The listing builds one solid part. Answer for the finished solid, in the listing's coordinates (mm). A direction names the side the tool comes from. Round coordinates to 2 decimals unless told otherwise and drop trailing zeros. Write each loop counter-clockwise with the first axis right and the second up, starting at its lowest first coordinate (ties: lowest second). Pieces come first, ordered by that corner, then holes.
Item 1: Find section D-D on x = 98. Give the vertices of the cut face in (y, z), then the cut area to 3 significant figures.
Item 2: Find section B-B on z = 34. Give the vertices of the cut face in (x, y).
Item 3: Find section A-A on y = 181.5. Give the vertices of the cut face in (x, z).
Item 4: Each of these flat-tipped pins is pushed along its axis until it touches: pin 1 (13.5 mm diameter, centred on y = 1118.5, z = 44.5, fed in from -X); pin 2 (2 mm diameter, centred on x = 269.5, y = 349.5, fed in from +Z); pin 3 (8.5 mm diameter, centred on x = 2.5, y = 389, fed in from -Z). Where does it stop, or does it pass through?
Item 5: For a pull along X with two mould halves and no side action, classify faces 4 (the face through (419.562, 740, 41)), 5 (the face through (204.3, 1500, 17.7)), 6 (the face through (217, 740, 18.133)) as +X half, -X half, draft (parallel to the pull), parting line (faces both ways), or undercut.
Item 6: Find section C-C on y = 993. Give the vertices of the cut face in (x, z), then the cut area to 4 significant figures.
Item 7: A tool of negligible diameter and unlimited length cuts with its end or side. For faces 1 (the face through (418.062, 740, 41)), 2 (the face through (9.562, 740, 41)), 3 (the face through (11.062, 740, 42)), from which of +Z, -Z, +X, -X, +Y, -Y can it reach the whole face along a straight path? Write none if from no direction.
Item 8: Find the intervals of material crossed by probe 1 along X at (y, z) = (796.5, 39); probe 2 along X at (y, z) = (339, 56); probe 3 along Z at (x, y) = (278.5, 337), in increasing order.
```python
from build123d import *

# Parameters (mm, degrees)
F1_DEPTH = 1500
F2_W     = 20
F2_H     = 100
F3_DEPTH = 1.5


with BuildPart() as f1:
    # F0 (on Front) → F1 (new body)
    with BuildSketch(Plane.XZ):
        Polygon((9.56153, 65.133369), (9.56153, 16.633369), (419.56153, 16.633369), (419.56153, 65.133369), (402.56153, 65.133369), (402.56153, 63.633369), (418.06153, 63.633369), (418.06153, 18.133369), (11.06153, 18.133369), (11.06153, 66.633369), (-8.93847, 66.633369), (-8.93847, 51.633369), (-7.43847, 51.633369), (-7.43847, 65.133369), align=None)
    extrude(amount=-F1_DEPTH)

    # F2 (on face) → F3 (cut, through all)
    with BuildSketch(Plane.XY.offset(18.133369)):
        with Locations((230.56153, 182)):
            Rectangle(F2_W, F2_H)
        with Locations((230.56153, 1307)):
            Rectangle(F2_W, F2_H)
    extrude(amount=-F3_DEPTH, mode=Mode.SUBTRACT)


solid = f1.part
```
Check values:
1. outline: (0, 16.63) - (1500, 16.63) - (1500, 18.13) - (0, 18.13) - close
1. area: 2,250 mm2
2. outline: (9.56, 0) - (11.06, 0) - (11.06, 1500) - (9.56, 1500) - close; (418.06, 0) - (419.56, 0) - (419.56, 1500) - (418.06, 1500) - close
3. outline: (-8.94, 51.63) - (-7.44, 51.63) - (-7.44, 65.13) - (9.56, 65.13) - (9.56, 16.63) - (220.56, 16.63) - (220.56, 18.13) - (11.06, 18.13) - (11.06, 66.63) - (-8.94, 66.63) - close; (240.56, 16.63) - (419.56, 16.63) - (419.56, 65.13) - (402.56, 65.13) - (402.56, 63.63) - (418.06, 63.63) - (418.06, 18.13) - (240.56, 18.13) - close
4. pin 1: stops at x = 9.56
4. pin 2: stops at z = 18.13
4. pin 3: stops at z = 65.13
5. face 4: +X half
5. face 5: draft
5. face 6: undercut
6. outline: (-8.94, 51.63) - (-7.44, 51.63) - (-7.44, 65.13) - (9.56, 65.13) - (9.56, 16.63) - (419.56, 16.63) - (419.56, 65.13) - (402.56, 65.13) - (402.56, 63.63) - (418.06, 63.63) - (418.06, 18.13) - (11.06, 18.13) - (11.06, 66.63) - (-8.94, 66.63) - close
6. area: 829.5 mm2
7. face 1: +Y, -Y
7. face 2: -Z, +Y, -Y
7. face 3: +Z, +Y, -Y
8. probe 1: x = 9.56 to 11.06, 418.06 to 419.56
8. probe 2: x = -8.94 to -7.44, 9.56 to 11.06, 418.06 to 419.56
8. probe 3: z = 16.63 to 18.13
